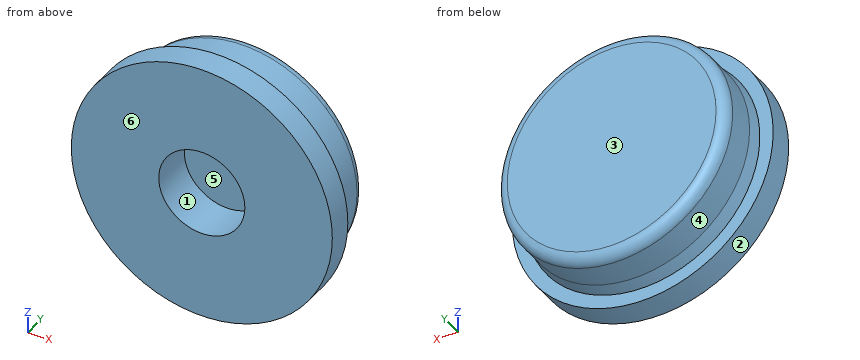
from build123d import *

# Parameters (mm, degrees)
SKETCH_2_R          = 5
EXTRUDE_1_DEPTH     = 1
SKETCH_3_R          = 4.4
EXTRUDE_2_DEPTH     = 2
FILLET_1_R          = 0.4
CHAMFER_1_SIZE      = 0.09
CHAMFER_1_SIZE2     = 0.510415364
SKETCH_4_R          = 1.65
CUT_EXTRUDE_1_DEPTH = 1.65


with BuildPart() as part:
    # 草图2 → 凸台-拉伸1 (new body)
    with BuildSketch(Plane(origin=(0, 0, 0), x_dir=(1, 0, 0), z_dir=(0, 1, 0))):
        Circle(SKETCH_2_R)
    extrude(amount=EXTRUDE_1_DEPTH)

    # 草图3 → 凸台-拉伸2 (add)
    with BuildSketch(Plane(origin=(0, 1, 0), x_dir=(1, 0, 0), z_dir=(0, 1, 0))):
        Circle(SKETCH_3_R)
    extrude(amount=EXTRUDE_2_DEPTH)

    # 圆角1
    fillet_1_edges = [part.edges().sort_by_distance(p)[0] for p in [
        (-4.4, 3, 0),
    ]]
    fillet(fillet_1_edges, radius=FILLET_1_R)

    # 倒角1
    chamfer_1_edges = [part.edges().sort_by_distance(p)[0] for p in [
        (-4.4, 1, 0),
    ]]
    chamfer_1_side = [part.faces().sort_by_distance(p)[0] for p in [
        (-4.858578644, 1, 0),
    ]]
    chamfer(chamfer_1_edges, length=CHAMFER_1_SIZE, length2=CHAMFER_1_SIZE2, reference=chamfer_1_side[0])

    # 草图4 → 切除-拉伸1 (cut)
    with BuildSketch(Plane.XZ):
        Circle(SKETCH_4_R)
    extrude(amount=-CUT_EXTRUDE_1_DEPTH, mode=Mode.SUBTRACT)


solid = part.part
The listing builds one solid part. Answer for the finished solid, in the listing's coordinates (mm). Face numbers are marked on the shaded views. A direction names the side the tool comes from. Round coordinates to 2 decimals unless told otherwise and drop trailing zeros. Order: outer loops, then holes, each group sorted by start corner. A loop starts at its lowest first (then second) coordinate and runs counter-clockwise, first axis right, second up. Notation, with made-up numbers: M 33,4.25 L 77,4.25 A11 ccw 77,23.25 Z; hole C -14.5,-29.75 d1. An arc over 180 degrees is marked long. Answer in a Markdown table with one row per item. Add a question column.
1) Consider line 1 along Z through (x, y) = (0, 0.75); line 2 along X through (y, z) = (0.8, 1.5); line 3 along Y through (x, z) = (2.75, 3.75). Determine where each line is inside the solid, lowest interval first. Write a range as from..to.
2) Determine the mould class of the marked faces 1, 2 and 3 for opening direction Z: pulls with the +Z half, pulls with the -Z half, needs draft (parallel to the pull), parting line crosses it, or undercut.
3) Flat-ended cylindrical pins translate along their axes: pin 1 Ø1 at (y, z) = (2, -1.5) entering from -X; pin 2 Ø1 at (x, y) = (-1, 1) entering from -Z; pin 3 Ø1.5 at (y, z) = (2, -0.5) entering from -X. Find the tip coordinate at first contact, or state that the pin passes through.
4) The part is cut by section D-D on y = 0.55. Determine the outline of the cut face in (x, z), plus the area to 3 significant figures.
5) The part is cut by section B-B on z = 0. Determine the outline of the cut face in (x, y).
6) The part is cut by section A-A on x = 0. Determine the outline of the cut face in (y, z), plus the area to 3 significant figures.
7) The part is cut by section C-C on y = 2.1. Determine the outline of the cut face in (x, z).
8) Which of the six approach directions +Z, -Z, +X, -X, +Y, -Y give full straight-line access (tool end or side, diameter ignored) to the marked faces 4, 5 and 6?
Findings below:
| question | item | result |
|---|---|---|
| 1 | line 1 | z = -5..-1.65, 1.65..5 |
| 1 | line 2 | x = -4.77..-0.69, 0.69..4.77 |
| 1 | line 3 | y = 0..1 |
| 2 | face 1 | undercut |
| 2 | face 2 | parting line crosses it |
| 2 | face 3 | needs draft |
| 3 | pin 1 | stops at x = -4.28 |
| 3 | pin 2 | stops at z = -4.97 |
| 3 | pin 3 | stops at x = -4.43 |
| 4 | outline | C 0,0 d10; hole C 0,0 d3.3 |
| 4 | area | 70.0 mm² |
| 5 | outline | M -5,0 L -1.65,0 L -1.65,1.65 L 1.65,1.65 L 1.65,0 L 5,0 L 5,1 L 4.49,1 L 4.4,1.51 L 4.4,2.6 A0.4 ccw 4,3 L -4,3 A0.4 ccw -4.4,2.6 L -4.4,1.51 L -4.49,1 L -5,1 Z |
| 6 | outline | M 0,-5 L 1,-5 L 1,-4.49 L 1.51,-4.4 L 2.6,-4.4 A0.4 ccw 3,-4 L 3,4 A0.4 ccw 2.6,4.4 L 1.51,4.4 L 1,4.49 L 1,5 L 0,5 L 0,1.65 L 1.65,1.65 L 1.65,-1.65 L 0,-1.65 Z |
| 6 | area | 22.1 mm² |
| 7 | outline | C 0,0 d8.8 |
| 8 | face 4 | +Y |
| 8 | face 5 | -Y |
| 8 | face 6 | +Z, -Z, +X, -X, -Y |
